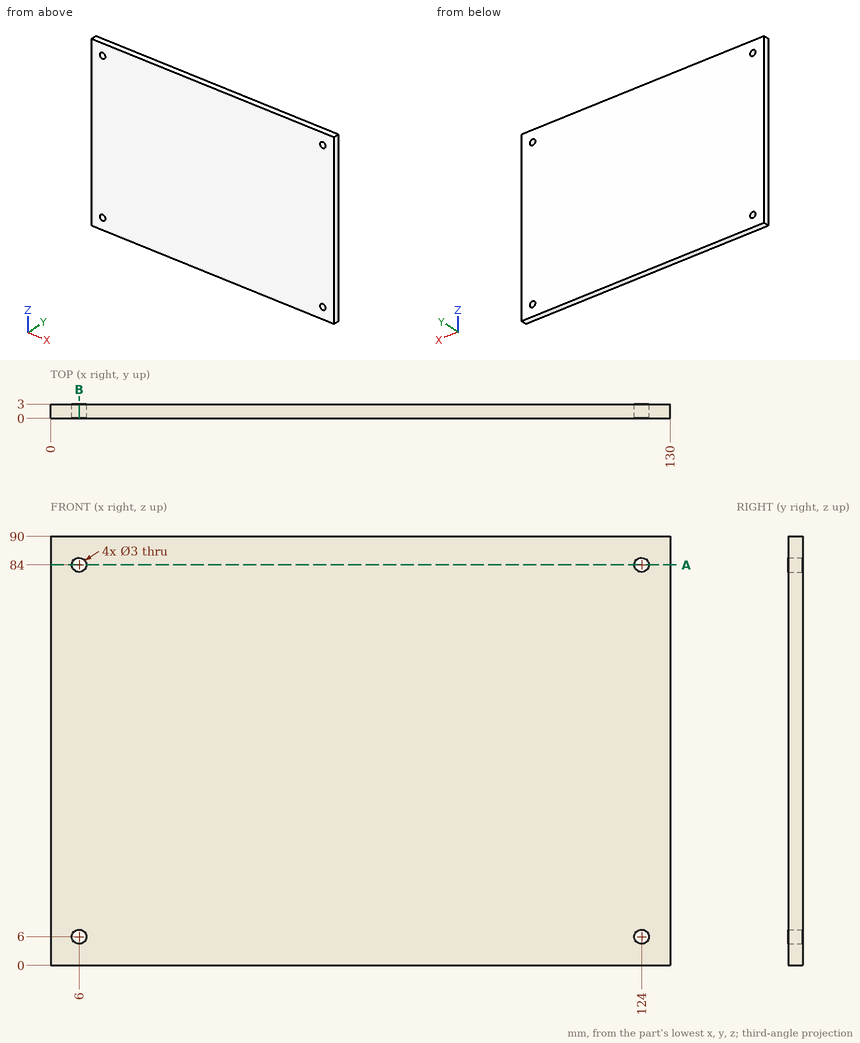
Check sheet for the drawn part. Datum: minimum x, y, z corner. Units: mm. Give positions to 0.01 mm unless a question says otherwise; leave off trailing zeros. Order: outer loops, then holes, each group sorted by start corner. A loop starts at its lowest first (then second) coordinate and runs counter-clockwise, first axis right, second up. Notation, with made-up numbers: (82.5, -15.75) - (102.5, -15.75) arc R27 ccw to (102.5, 6.25) - close; hole circle Ø11 at (56.25, 18.25). An arc over 180 degrees is marked (long way). Answer as a JSON object with one key per item and string values.
(1) Cross-section at A-A (z = 84). Record the cut outline in (x, y).
Report:
{"outline": "(0, 0) - (4.5, 0) - (4.5, 3) - (0, 3) - close; (7.5, 0) - (122.5, 0) - (122.5, 3) - (7.5, 3) - close; (125.5, 0) - (130, 0) - (130, 3) - (125.5, 3) - close"}
(2) Cross-section at B-B (x = 6). Record the cut outline in (y, z), then the cut area to 3 significant figures.
Report:
{"outline": "(0, 0) - (3, 0) - (3, 4.5) - (0, 4.5) - close; (0, 7.5) - (3, 7.5) - (3, 82.5) - (0, 82.5) - close; (0, 85.5) - (3, 85.5) - (3, 90) - (0, 90) - close", "area": "252 mm^2"}
(3) Material ranges on line 1 (X direction, y = 1.3, z = 6); line 2 (Z direction, x = 6, y = 2.15), recorded low to high.
Report:
{"line 1": "0 to 4.5, 7.5 to 122.5, 125.5 to 130", "line 2": "0 to 4.5, 7.5 to 82.5, 85.5 to 90"}
